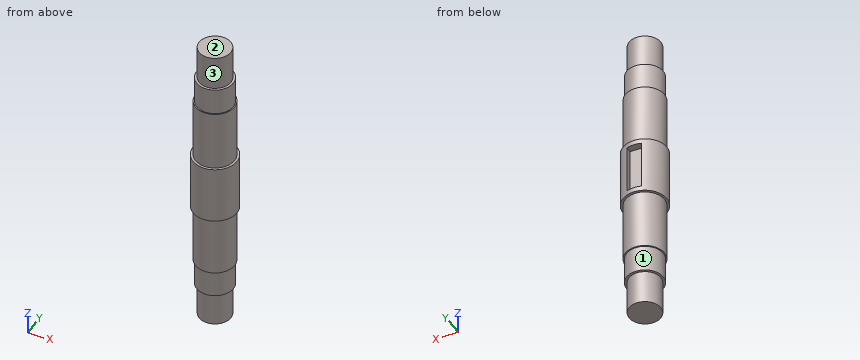
from build123d import *

# Parameters (mm, degrees)
SKETCH1_R           = 6.5
BOSS_EXTRUDE1_DEPTH = 14
SKETCH2_R           = 7.5
BOSS_EXTRUDE2_DEPTH = 11
SKETCH3_R           = 8
BOSS_EXTRUDE3_DEPTH = 25
SKETCH4_R           = 9
BOSS_EXTRUDE4_DEPTH = 12
SKETCH5_W           = 6
SKETCH5_H           = 20
CUT_EXTRUDE2_DEPTH  = 3


with BuildPart() as part:
    # Sketch1 → Boss-Extrude1 (new body)
    with BuildSketch(Plane(origin=(0, 0, 0), x_dir=(0, 1, 0), z_dir=(0, 0, 1))):
        with Locations(Location((0, 0, 0), (0, 0, 270))):
            Circle(SKETCH1_R)
    extrude(amount=BOSS_EXTRUDE1_DEPTH)

    # Sketch2 → Boss-Extrude2 (add)
    with BuildSketch(Plane.XY.offset(14)):
        Circle(SKETCH2_R)
    extrude(amount=BOSS_EXTRUDE2_DEPTH)

    # Sketch3 → Boss-Extrude3 (add)
    with BuildSketch(Plane.XY.offset(25)):
        Circle(SKETCH3_R)
    extrude(amount=BOSS_EXTRUDE3_DEPTH)

    # Sketch4 → Boss-Extrude4 (add)
    with BuildSketch(Plane.XY.offset(50)):
        Circle(SKETCH4_R)
    extrude(amount=BOSS_EXTRUDE4_DEPTH)

    # Mirror1: part across plane


with BuildPart() as part_1:
    add(part.part)
    add(part.part.mirror(Plane.XY.offset(62)))

    # Sketch5 → Cut-Extrude2 (cut)
    with BuildSketch(Plane(origin=(0, 9, 0), x_dir=(-1, 0, 0), z_dir=(0, 1, 0))):
        with Locations((0, 62)):
            Rectangle(SKETCH5_W, SKETCH5_H)
    extrude(amount=-CUT_EXTRUDE2_DEPTH, mode=Mode.SUBTRACT)


solid = part_1.part
The listing builds one solid part. Answer for the finished solid, in the listing's coordinates (mm). Face numbers are marked on the shaded views. A direction names the side the tool comes from. Coordinates: 2 decimals unless noted, no trailing zeros. Write each loop counter-clockwise with the first axis right and the second up, starting at its lowest first coordinate (ties: lowest second). Pieces come first, ordered by that corner, then holes. Notation, with made-up numbers: (59, 26.5) - (64, 26.5) arc R12 ccw to (64, 39.5) - close; hole circle Ø4 at (38, -18.5). An arc over 180 degrees is marked (long way). Put each result on its own line as item: value.
1. The part is cut by section A-A on y = 0. Give the vertices of the cut face in (x, z), plus the area to 3 significant figures.
Answer sheet:
outline: (-9, 50) - (-8, 50) - (-8, 25) - (-7.5, 25) - (-7.5, 14) - (-6.5, 14) - (-6.5, 0) - (6.5, 0) - (6.5, 14) - (7.5, 14) - (7.5, 25) - (8, 25) - (8, 50) - (9, 50) - (9, 74) - (8, 74) - (8, 99) - (7.5, 99) - (7.5, 110) - (6.5, 110) - (6.5, 124) - (-6.5, 124) - (-6.5, 110) - (-7.5, 110) - (-7.5, 99) - (-8, 99) - (-8, 74) - (-9, 74) - close
area: 1,930 mm^2
2. The part is cut by section D-D on x = -4.75. Give the vertices of the cut face in (y, z).
Answer sheet:
outline: (-7.64, 50) - (-6.44, 50) - (-6.44, 25) - (-5.8, 25) - (-5.8, 14) - (-4.44, 14) - (-4.44, 0) - (4.44, 0) - (4.44, 14) - (5.8, 14) - (5.8, 25) - (6.44, 25) - (6.44, 50) - (7.64, 50) - (7.64, 74) - (6.44, 74) - (6.44, 99) - (5.8, 99) - (5.8, 110) - (4.44, 110) - (4.44, 124) - (-4.44, 124) - (-4.44, 110) - (-5.8, 110) - (-5.8, 99) - (-6.44, 99) - (-6.44, 74) - (-7.64, 74) - close
3. Flat-ended cylindrical pins translate along their axes: pin 1 Ø8 at (y, z) = (-1.5, 18) entering from -X; pin 2 Ø5 at (x, z) = (0.5, 32.5) entering from -Y; pin 3 Ø5 at (y, z) = (5, 39) entering from -X. Find the tip coordinate at first contact, or state that the pin passes through.
Answer sheet:
pin 1: stops at x = -7.5
pin 2: stops at y = -8
pin 3: stops at x = -7.6
4. A tool of negligible diameter and unlimited length cuts with its end or side. For the marked faces 1, 2 and 3, from which of +Z, -Z, +X, -X, +Y, -Y can it reach the whole face along a straight path? Write none if from no direction.
Answer sheet:
face 1: -Z
face 2: +Z, +X, -X, +Y, -Y
face 3: +Z
5. Find the intervals of material crossed by line 1 along Z through (x, y) = (2.75, 6.25); line 2 along Y through (x, z) = (-3.75, 104); line 3 along Y through (x, z) = (2.75, 94.5), in increasing order. Write a range as from..to.
Answer sheet:
line 1: z = 14..52, 72..110
line 2: y = -6.5..6.5
line 3: y = -7.51..7.51
6. The part is cut by section C-C on z = 104.5. Give the vertices of the cut face in (x, y).
Answer sheet:
outline: circle Ø15 at (0, 0)
